Could you check a few things on this model? Use its own coordinates, in mm. Round coordinates to 2 decimals unless told otherwise and drop trailing zeros. Write each loop counter-clockwise with the first axis right and the second up, starting at its lowest first coordinate (ties: lowest second). Pieces come first, ordered by that corner, then holes. Notation, with made-up numbers: (29.5, 41.5) - (42.5, 41.5) arc R10 ccw to (42.5, 59.5) - close; hole circle Ø8 at (30, 59.5). An arc over 180 degrees is marked (long way). Put each result on its own line as item: value.
from build123d import *

# Parameters (mm, degrees)
F0_R     = 6.5
F0_R_2   = 2
F0_R_3   = 3
F0_R_4   = 9
F1_DEPTH = 7


with BuildPart() as f1:
    # F0 (on Right) → F1 (new body)
    with BuildSketch(Plane.YZ):
        with BuildLine():
            Line((55, -5), (58, 0))
            Line((58, 0), (87, 0))
            Line((87, 0), (87, 8))
            ThreePointArc((87, 8), (97, 18), (107, 8))
            Line((107, 8), (107, 0))
            Line((107, 0), (136, 0))
            Line((136, 0), (136, 40))
            Line((136, 40), (143, 40))
            Line((143, 40), (143, 48))
            Line((143, 48), (136, 48))
            Line((136, 48), (136, 53))
            Line((136, 53), (130, 53))
            Line((130, 53), (130, 52))
            Line((130, 52), (127, 52))
            Line((127, 52), (127, 53))
            Line((127, 53), (122, 53))
            Line((122, 53), (122, 55))
            Line((122, 55), (122, 57))
            Line((122, 57), (127, 57))
            Line((127, 57), (127, 58))
            Line((127, 58), (130, 58))
            Line((130, 58), (130, 57))
            Line((130, 57), (136, 57))
            Line((136, 57), (136, 62))
            Line((136, 62), (143, 62))
            Line((143, 62), (143, 70))
            Line((143, 70), (136, 70))
            Line((136, 70), (136, 86))
            Line((136, 86), (130, 86))
            Line((130, 86), (130, 85))
            Line((130, 85), (127, 85))
            Line((127, 85), (127, 86))
            Line((127, 86), (122, 86))
            Line((122, 86), (122, 88))
            Line((122, 88), (122, 90))
            Line((122, 90), (127, 90))
            Line((127, 90), (127, 91))
            Line((127, 91), (130, 91))
            Line((130, 91), (130, 90))
            Line((130, 90), (136, 90))
            Line((136, 90), (136, 101))
            Line((136, 101), (130, 101))
            Line((130, 101), (130, 100))
            Line((130, 100), (127, 100))
            Line((127, 100), (127, 101))
            Line((127, 101), (122, 101))
            Line((122, 101), (122, 103))
            Line((122, 103), (122, 105))
            Line((122, 105), (127, 105))
            Line((127, 105), (127, 106))
            Line((127, 106), (130, 106))
            Line((130, 106), (130, 105))
            Line((130, 105), (136, 105))
            Line((136, 105), (136, 358))
            Line((136, 358), (143, 358))
            Line((143, 358), (143, 366))
            Line((143, 366), (136, 366))
            Line((136, 366), (136, 371))
            Line((136, 371), (130, 371))
            Line((130, 371), (130, 370))
            Line((130, 370), (127, 370))
            Line((127, 370), (127, 371))
            Line((127, 371), (122, 371))
            Line((122, 371), (122, 373))
            Line((122, 373), (122, 375))
            Line((122, 375), (127, 375))
            Line((127, 375), (127, 376))
            Line((127, 376), (130, 376))
            Line((130, 376), (130, 375))
            Line((130, 375), (136, 375))
            Line((136, 375), (136, 380))
            Line((136, 380), (143, 380))
            Line((143, 380), (143, 388))
            Line((143, 388), (136, 388))
            Line((136, 388), (136, 401))
            Line((136, 401), (122, 401))
            Line((122, 401), (122, 395))
            Line((122, 395), (123, 395))
            Line((123, 395), (123, 392))
            Line((123, 392), (122, 392))
            Line((122, 392), (122, 387))
            Line((122, 387), (120, 387))
            Line((120, 387), (118, 387))
            Line((118, 387), (118, 392))
            Line((118, 392), (117, 392))
            Line((117, 392), (117, 395))
            Line((117, 395), (118, 395))
            Line((118, 395), (118, 401))
            Line((118, 401), (112, 401))
            Line((112, 401), (112, 408))
            Line((112, 408), (97, 408))
            Line((97, 408), (97, 401))
            Line((97, 401), (92, 401))
            Line((92, 401), (0, 55))
            Line((0, 55), (0, 41))
            Line((0, 41), (6, 41))
            Line((6, 41), (6, 42))
            Line((6, 42), (9, 42))
            Line((9, 42), (9, 41))
            Line((9, 41), (14, 41))
            Line((14, 41), (14, 39))
            Line((14, 39), (14, 37))
            Line((14, 37), (9, 37))
            Line((9, 37), (9, 36))
            Line((9, 36), (6, 36))
            Line((6, 36), (6, 37))
            Line((6, 37), (0, 37))
            Line((0, 37), (0, 33))
            Line((0, 33), (-7, 33))
            Line((-7, 33), (-7, 23))
            Line((-7, 23), (-7, 13))
            Line((-7, 13), (0, 13))
            Line((0, 13), (0, 9))
            Line((0, 9), (6, 9))
            Line((6, 9), (6, 10))
            Line((6, 10), (9, 10))
            Line((9, 10), (9, 9))
            Line((9, 9), (14, 9))
            Line((14, 9), (14, 7))
            Line((14, 7), (14, 5))
            Line((14, 5), (9, 5))
            Line((9, 5), (9, 4))
            Line((9, 4), (6, 4))
            Line((6, 4), (6, 5))
            Line((6, 5), (0, 5))
            Line((0, 5), (0, 0))
            Line((0, 0), (0, -5))
            Line((0, -5), (55, -5))
        make_face()
        with Locations((28.5, 14.5)):
            Circle(F0_R, mode=Mode.SUBTRACT)
        with Locations((112, 28)):
            Circle(F0_R_2, mode=Mode.SUBTRACT)
        with BuildLine():
            ThreePointArc((57.29765, 134.284836), (59.082144, 136.963848), (62.129751, 138))
            Line((62.129751, 138), (96, 138))
            ThreePointArc((96, 138), (99.535534, 136.535534), (101, 133))
            Line((101, 133), (101, 65))
            ThreePointArc((101, 65), (99.535534, 61.464466), (96, 60))
            Line((96, 60), (44.048826, 60))
            ThreePointArc((44.048826, 60), (40.084978, 61.952393), (39.216725, 66.284836))
            Line((39.216725, 66.284836), (57.29765, 134.284836))
        make_face(mode=Mode.SUBTRACT)
        with BuildLine():
            Line((101, 223), (101, 153))
            Line((101, 153), (61, 153))
            Line((61, 153), (80.27254, 225.481509))
            ThreePointArc((80.27254, 225.481509), (91.713641, 233.239781), (101, 223))
        make_face(mode=Mode.SUBTRACT)
        with Locations((112, 112)):
            Circle(F0_R_2, mode=Mode.SUBTRACT)
        with Locations((112, 132)):
            Circle(F0_R_2, mode=Mode.SUBTRACT)
        with Locations((70, 232)):
            Circle(F0_R_2, mode=Mode.SUBTRACT)
        with Locations((95.884576, 265.975365)):
            Circle(F0_R_2, mode=Mode.SUBTRACT)
        with Locations((112, 232)):
            Circle(F0_R_2, mode=Mode.SUBTRACT)
        with Locations((112, 316)):
            Circle(F0_R_2, mode=Mode.SUBTRACT)
        with Locations((112, 325)):
            Circle(F0_R_3, mode=Mode.SUBTRACT)
        with Locations((112, 342)):
            Circle(F0_R_4, mode=Mode.SUBTRACT)
        with Locations((112, 356)):
            Circle(F0_R_2, mode=Mode.SUBTRACT)
    extrude(amount=F1_DEPTH)


solid = f1.part
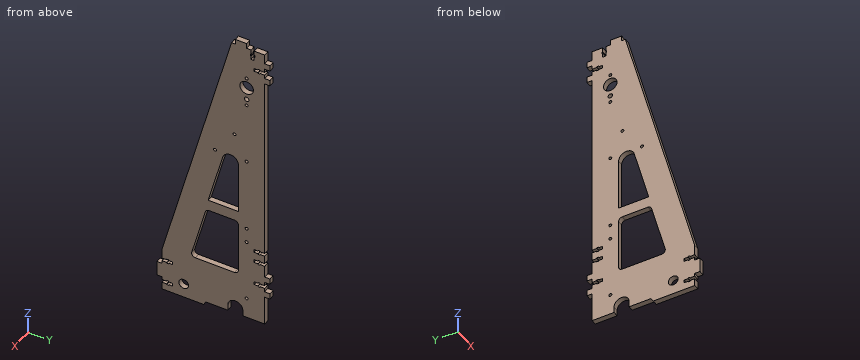
(1) Imagine slicing it at B-B, the plane y = 28.5. List the corners of the cut face in (x, z) for me, then the cut area to 3 significant figures.
Values found:
outline: (0, -5) - (7, -5) - (7, 8) - (0, 8) - close; (0, 21) - (7, 21) - (7, 162.18) - (0, 162.18) - close
area: 1,080 mm^2
(2) Imagine slicing it at D-D, the plane z = 289.5. List the corners of the cut face in (x, y) for me.
Values found:
outline: (0, 62.35) - (7, 62.35) - (7, 136) - (0, 136) - close
(3) Imagine slicing it at C-C, the plane x = 1.25. Give the number of separate pieces and of enclosed holes in the cut face, then the cut area to 3 significant figures.
Values found:
separate pieces: 1
enclosed holes: 13
area: 31,700 mm^2
(4) Imagine slicing it at A-A, the plane z = 342. List the corners of the cut face in (x, y) for me.
Values found:
outline: (0, 76.31) - (7, 76.31) - (7, 103) - (0, 103) - close; (0, 121) - (7, 121) - (7, 136) - (0, 136) - close
(5) I'm going to push flat-ended pins straight in: pin 1 (12 mm diameter, centred on y = 10, z = 129, fed in from -X); pin 2 (1.1 mm diameter, centred on x = 4.5, z = 370.5, fed in from -Y); pin 3 (3.5 mm diameter, centred on x = 3, z = 391.5, fed in from +Y); pin 4 (3 mm diameter, centred on x = 2, z = 79, fed in from -Y). Where does each tip first touch, or does it pass through?
Values found:
pin 1: passes through
pin 2: stops at y = 83.74
pin 3: stops at y = 136
pin 4: stops at y = 5.98
(6) Please list where these lines run through material, in increasing order: probe 1 along Z at (x, y) = (5.5, 131); probe 2 along Y at (x, z) = (0.5, 36.5); probe 3 along Y at (x, z) = (2.5, 232). Write a range as from..to.
Values found:
probe 1: z = 0..53, 57..86, 90..101, 105..371, 375..401
probe 2: y = 0..6, 9..136
probe 3: y = 47.06..68, 72..85.36, 95.56..110, 114..136
